Can you work these out from the drawing? Everything is in mm from the part's minimum corner. A direction names the side the tool comes from. Round coordinates to 2 decimals unless told otherwise and drop trailing zeros. Order: outer loops, then holes, each group sorted by start corner. A loop starts at its lowest first (then second) coordinate and runs counter-clockwise, first axis right, second up. Notation, with made-up numbers: (-21, -29.75) -> (12, -29.75) arc R31 cw to (12, 3.25) -> close; hole circle Ø11 at (26, -24). An arc over 180 degrees is marked (long way). One line per item, written item: value.
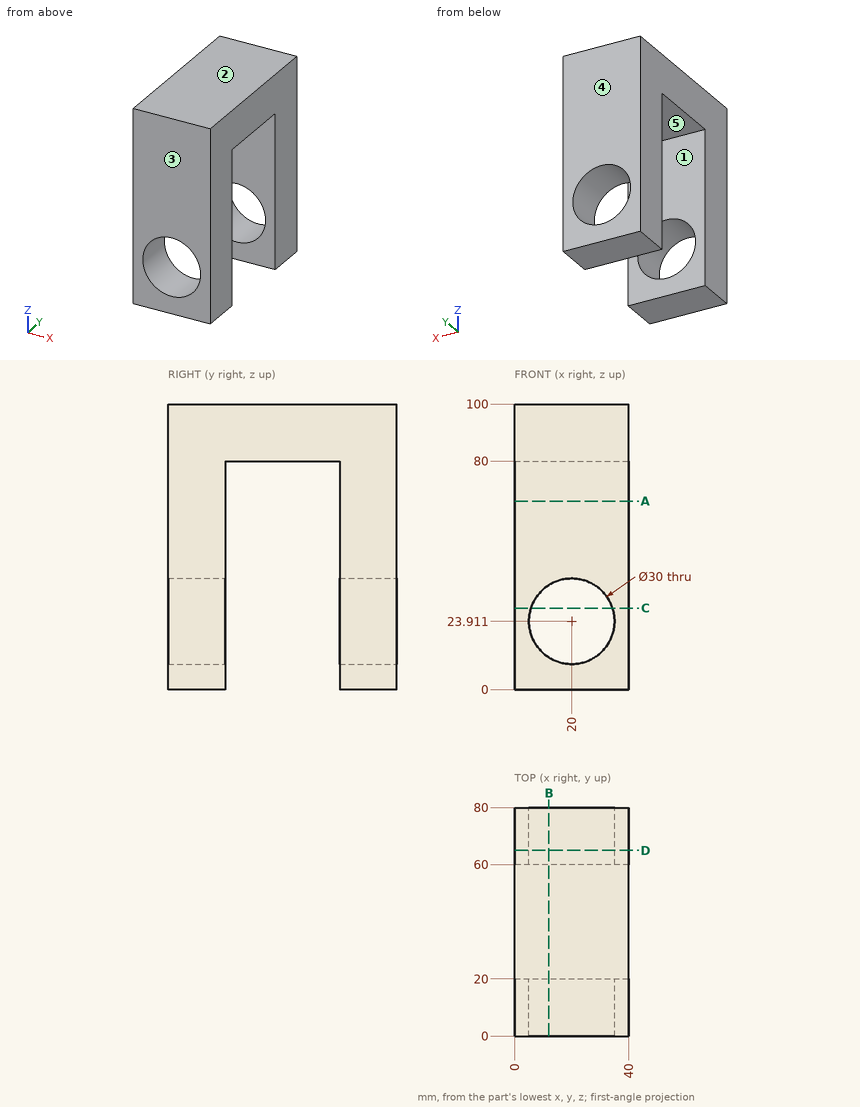
Q1. Will this pin go through, and if not, where does the flat tip stop? pin 1 Ø20 at (x, y) = (20.5, 37.5) entering from -Z.
Answers below:
pin 1: z = 80
Q2. We'd pull the mould along Y, two halves only. Please class the marked faces 1, 2 and 3: released by +Y, released by -Y, zero draft, split by the parting line, or undercut.
Answers below:
face 1: undercut
face 2: zero draft
face 3: released by -Y
Q3. On a 3-axis mill with a long thin cutter (end or side, diameter ignored), from which of +Z, -Z, +X, -X, +Y, -Y can I reach the whole of each face in a straight line? I mean the marked faces 4 and 5. Say none if no direction works.
Answers below:
face 4: +Z, -Z, +X, -X, +Y
face 5: -Z, +X, -X
Q4. I want a section at B-B on x = 12. List the corners of the cut face in (y, z) for me.
Answers below:
outline: (0, 0) -> (20, 0) -> (20, 11.22) -> (0, 11.22) -> close; (0, 36.6) -> (20, 36.6) -> (20, 80) -> (60, 80) -> (60, 36.6) -> (80, 36.6) -> (80, 100) -> (0, 100) -> close; (60, 0) -> (80, 0) -> (80, 11.22) -> (60, 11.22) -> close
Q5. I want a section at C-C on z = 28.5. List the corners of the cut face in (x, y) for me.
Answers below:
outline: (0, 0) -> (5.72, 0) -> (5.72, 20) -> (0, 20) -> close; (0, 60) -> (5.72, 60) -> (5.72, 80) -> (0, 80) -> close; (34.28, 0) -> (40, 0) -> (40, 20) -> (34.28, 20) -> close; (34.28, 60) -> (40, 60) -> (40, 80) -> (34.28, 80) -> close
Q6. Please list where these lines run through material, in increasing order: line 1 along Y through (x, z) = (13.5, 45.5); line 2 along Z through (x, y) = (20, 75); line 3 along Z through (x, y) = (14.5, 38.5).
Answers below:
line 1: 0 to 20, 60 to 80
line 2: 0 to 8.91, 38.91 to 100
line 3: 80 to 100
Q7. I want a section at A-A on z = 66. List the corners of the cut face in (x, y) for me, plus the area to 3 significant figures.
Answers below:
outline: (0, 0) -> (40, 0) -> (40, 20) -> (0, 20) -> close; (0, 60) -> (40, 60) -> (40, 80) -> (0, 80) -> close
area: 1,600 mm^2
Q8. I want a section at D-D on y = 65. List the corners of the cut face in (x, z) for me.
Answers below:
outline: (0, 0) -> (40, 0) -> (40, 100) -> (0, 100) -> close; hole circle Ø30 at (20, 23.91)
